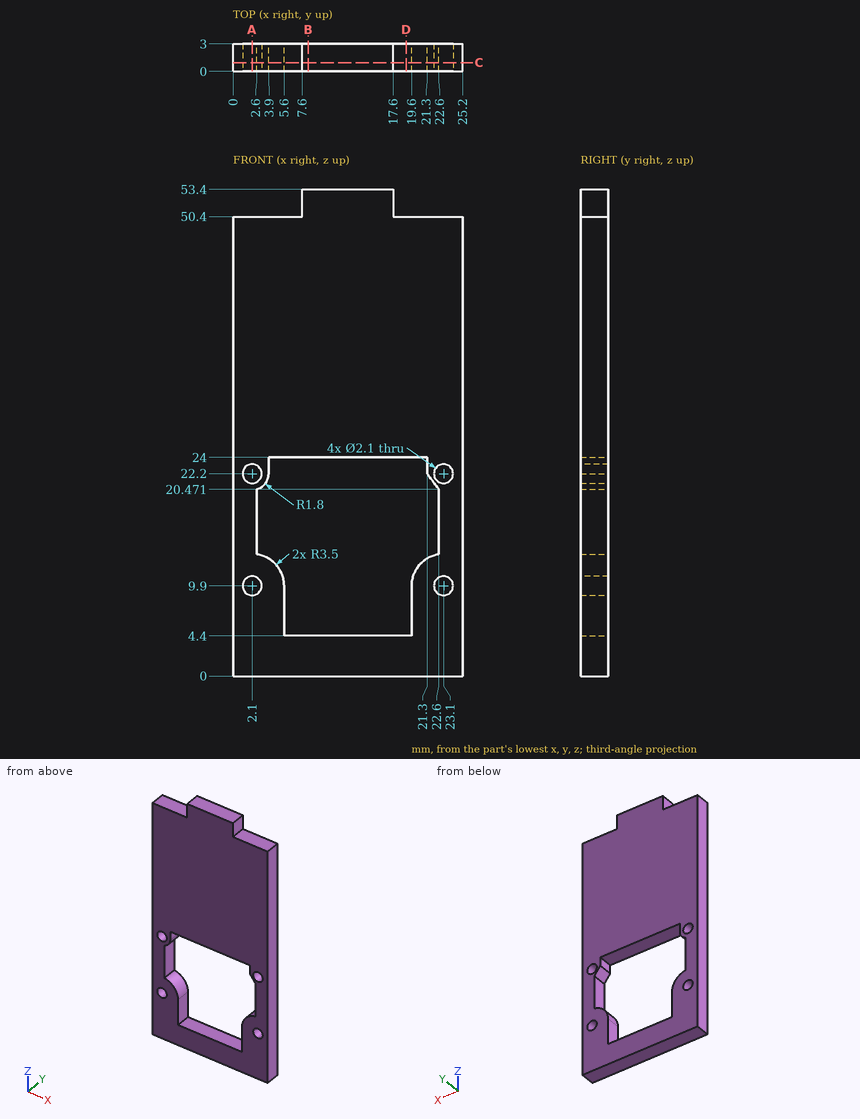
Check sheet for the drawn part. Datum: minimum x, y, z corner. Units: mm. Coordinates: 2 decimals unless noted, no trailing zeros. Loops run counter-clockwise (first coordinate to the right, second up) from the corner with the lowest first, then second, coordinate; pieces in that order, holes last. Notation, with made-up numbers: (63, 73) -> (99, 73) arc R17 cw to (99, 96) -> close; hole circle Ø10 at (42, 34.5). An arc over 180 degrees is marked (long way). Write each question's results on one line, items separated by ' | '.
Item 1: Section check A-A, the plane x = 2.1. Enter the section's corners in (y, z), plus the area to 3 significant figures.
Found:
outline: (0, 0) -> (3, 0) -> (3, 8.85) -> (0, 8.85) -> close; (0, 10.95) -> (3, 10.95) -> (3, 21.15) -> (0, 21.15) -> close; (0, 23.25) -> (3, 23.25) -> (3, 50.4) -> (0, 50.4) -> close | area: 139 mm2
Item 2: Section check D-D, the plane x = 19. Enter the section's corners in (y, z).
Found:
outline: (0, 0) -> (3, 0) -> (3, 4.4) -> (0, 4.4) -> close; (0, 24) -> (3, 24) -> (3, 50.4) -> (0, 50.4) -> close
Item 3: Gauge pin test, flat ends, axial feed: pin 1 (1 mm diameter, centred on x = 21, y = 0.5, fed in from +Z); pin 2 (1.7 mm diameter, centred on x = 23.1, z = 9.9, fed in from +Y). Record the tip position at first contact, or that the pin passes through.
Found:
pin 1: stops at z = 50.4 | pin 2: passes through
Item 4: Section check C-C, the plane y = 0.95. Enter the section's corners in (x, z).
Found:
outline: (0, 0) -> (25.2, 0) -> (25.2, 50.4) -> (17.6, 50.4) -> (17.6, 53.4) -> (7.6, 53.4) -> (7.6, 50.4) -> (0, 50.4) -> close; hole circle Ø2.1 at (2.1, 9.9); hole circle Ø2.1 at (2.1, 22.2); hole (2.6, 13.36) arc R3.5 cw to (5.6, 9.9) -> (5.6, 4.4) -> (19.6, 4.4) -> (19.6, 9.9) arc R3.5 cw to (22.6, 13.36) -> (22.6, 20.47) -> (21.3, 22.2) -> (21.3, 24) -> (3.9, 24) -> (3.9, 22.2) arc R1.8 cw to (2.6, 20.47) -> close; hole circle Ø2.1 at (23.1, 9.9); hole circle Ø2.1 at (23.1, 22.2)
Item 5: Section check B-B, the plane x = 8.25. Enter the section's corners in (y, z).
Found:
outline: (0, 0) -> (3, 0) -> (3, 4.4) -> (0, 4.4) -> close; (0, 24) -> (3, 24) -> (3, 53.4) -> (0, 53.4) -> close
Item 6: Material ranges on L1, parallel to Z at x = 23.1, y = 1.9; L2, parallel to X at y = 1.1, z = 9.9; L3, parallel to X at y = 0.95, z = 22.2, recorded low to high.
Found:
L1: z = 0 to 8.85, 10.95 to 21.15, 23.25 to 50.4 | L2: x = 0 to 1.05, 3.15 to 5.6, 19.6 to 22.05, 24.15 to 25.2 | L3: x = 0 to 1.05, 3.15 to 3.9, 21.3 to 22.05, 24.15 to 25.2
